Build history of the part. All positions in model axes, mm. A direction names the side the tool comes from. Give positions to 0.01 mm unless a question says otherwise; leave off trailing zeros. Order: outer loops, then holes, each group sorted by start corner. A loop starts at its lowest first (then second) coordinate and runs counter-clockwise, first axis right, second up. Notation, with made-up numbers: M -10.5,33.5 L 3.5,33.5 A25 cw 3.5,70.5 Z; hole C 1.5,29.5 d8. An arc over 180 degrees is marked long. One line per item, written item: value. Start each with the question number.
from build123d import *
from build123d.topology import SkipClean

# Parameters (mm, degrees)
SKETCH1_R               = 7.5
BOSS_EXTRUDE1_DEPTH     = 6.779166667
SKETCH1_3_R             = 7.5
BOSS_EXTRUDE2_DEPTH     = 2.779166667
BOSS_EXTRUDE3_START     = -4
SKETCH1_4_R             = 7.5
BOSS_EXTRUDE3_DEPTH     = 4
SKETCH2_R               = 5
BOSS_EXTRUDE4_DEPTH     = 6.016666667
SKETCH2_3_R             = 5.5
SKETCH2_3_R_2           = 5
BOSS_EXTRUDE5_DEPTH     = 1.254166667
BOSS_EXTRUDE9_START     = 16.541666667
SKETCH3_R               = 5
BOSS_EXTRUDE9_DEPTH     = 16.541666667
BOSS_EXTRUDE10_START    = 12.541666667
SKETCH3_3_R             = 5.5
SKETCH3_3_R_2           = 5
BOSS_EXTRUDE10_DEPTH    = 12.541666667
BOSS_EXTRUDE11_DEPTH    = 9.4
CUT_EXTRUDE1_DEPTH      = 28.502022969
CUT_EXTRUDE1_DEPTH_BACK = 28.502022969
SKETCH5_R               = 1.575
CUT_EXTRUDE5_START      = -2.779166667
CUT_EXTRUDE5_DEPTH      = 2.779166667
BOSS_EXTRUDE12_START    = -2.779166667
SKETCH6_4_R             = 9
BOSS_EXTRUDE12_DEPTH    = 2.779166667


with BuildPart() as part:
    # Sketch1 → Boss-Extrude1 (new body)
    with BuildSketch(Plane(origin=(0, 0, 0), x_dir=(1, 0, 0), z_dir=(0, 1, 0))):
        with Locations(Location((-1, 0, 0), (0, 0, 270))):
            Circle(SKETCH1_R)
    extrude(amount=BOSS_EXTRUDE1_DEPTH)

    # Sketch1<3> → Boss-Extrude2 (add)
    with BuildSketch(Plane(origin=(0, 0, 0), x_dir=(1, 0, 0), z_dir=(0, 1, 0))):
        with Locations(Location((-1, 0, 0), (0, 0, 82.337744339))):
            Circle(SKETCH1_3_R)
        with Locations((1, 0)):
            Circle(SKETCH1_3_R)
    extrude(amount=BOSS_EXTRUDE2_DEPTH)

    # Sketch1<4> → Boss-Extrude3 (add)
    with BuildSketch(Plane(origin=(0, 0, 0), x_dir=(1, 0, 0), z_dir=(0, 1, 0)).offset(BOSS_EXTRUDE3_START)):
        with Locations(Location((1, 0, 0), (0, 0, 97.662255661))):
            Circle(SKETCH1_4_R)
        with BuildLine():
            Line((-1.54175225, 2.127), (1.54175225, 2.127))
            ThreePointArc((1.54175225, 2.127), (0, -2.627), (-1.54175225, 2.127))
        make_face(mode=Mode.SUBTRACT)
    extrude(amount=BOSS_EXTRUDE3_DEPTH)

    # Sketch2 → Boss-Extrude4 (add)
    with BuildSketch(Plane.XZ.offset(4)):
        with Locations(Location((0, 0, 0), (0, 0, 90))):
            Circle(SKETCH2_R)
    extrude(amount=BOSS_EXTRUDE4_DEPTH)

    # Sketch2<3> → Boss-Extrude5 (add)
    with BuildSketch(Plane.XZ.offset(4)):
        with Locations(Location((0, 0, 0), (0, 0, 90))):
            Circle(SKETCH2_3_R)
        with Locations(Location((0, 0, 0), (0, 0, 270))):
            Circle(SKETCH2_3_R_2, mode=Mode.SUBTRACT)
    extrude(amount=BOSS_EXTRUDE5_DEPTH)

    # Sketch3 → Boss-Extrude9 (add)
    with BuildSketch(Plane(origin=(0, 6.779166667, 0), x_dir=(1, 0, 0), z_dir=(0, 1, 0)).offset(BOSS_EXTRUDE9_START)):
        with Locations(Location((0, 0, 0), (0, 0, 90))):
            Circle(SKETCH3_R)
    extrude(amount=-BOSS_EXTRUDE9_DEPTH)

    # Sketch3<3> → Boss-Extrude10 (add)
    with BuildSketch(Plane(origin=(0, 6.779166667, 0), x_dir=(1, 0, 0), z_dir=(0, 1, 0)).offset(BOSS_EXTRUDE10_START)):
        with Locations(Location((0, 0, 0), (0, 0, 270))):
            Circle(SKETCH3_3_R)
        with Locations(Location((0, 0, 0), (0, 0, 90))):
            Circle(SKETCH3_3_R_2, mode=Mode.SUBTRACT)
    extrude(amount=-BOSS_EXTRUDE10_DEPTH)

    # Sketch4 → Boss-Extrude11 (add)
    with BuildSketch(Plane.XZ.offset(10.016666667)):
        with BuildLine():
            Line((-4, 3), (-4, -3))
            ThreePointArc((-4, -3), (0, -5), (4, -3))
            Line((4, -3), (4, 3))
            ThreePointArc((4, 3), (0, 5), (-4, 3))
        make_face()
    extrude(amount=BOSS_EXTRUDE11_DEPTH)

    # Sketch5 → Cut-Extrude1 (cut, two sides: drawn at the far end of the back side and taken through both)
    with BuildSketch(Plane(origin=(4, 0, 0), x_dir=(0, 0, -1), z_dir=(1, 0, 0)).offset(-CUT_EXTRUDE1_DEPTH_BACK)):
        with Locations(Location((-1.35, -16.416666667, 0), (0, 0, 180))):
            Circle(SKETCH5_R)
        with Locations(Location((1.35, -13.416666667, 0), (0, 0, 180))):
            Circle(SKETCH5_R)
    extrude(amount=CUT_EXTRUDE1_DEPTH + CUT_EXTRUDE1_DEPTH_BACK, mode=Mode.SUBTRACT)

    # Sketch6 → Cut-Extrude5 (cut)
    with SkipClean():  # the faces are left unmerged after this step: merging them gives an invalid solid
        with BuildSketch(Plane(origin=(0, 2.779166667, 0), x_dir=(1, 0, 0), z_dir=(0, 1, 0)).offset(CUT_EXTRUDE5_START)):
            with BuildLine():
                ThreePointArc((0, -7.433034374), (8.5, 0), (0, 7.433034374))
                ThreePointArc((0, 7.433034374), (6.5, 0), (0, -7.433034374))
            make_face()
        extrude(amount=CUT_EXTRUDE5_DEPTH, mode=Mode.SUBTRACT)

    # Sketch6<4> → Boss-Extrude12 (add)
    # profile 1 of 2: a face of its own
    with BuildSketch(Plane(origin=(0, 2.779166667, 0), x_dir=(1, 0, 0), z_dir=(0, 1, 0)).offset(BOSS_EXTRUDE12_START)):
        with Locations(Location((0, 0, 0), (0, 0, 270))):
            Circle(SKETCH6_4_R)
        with BuildLine():
            ThreePointArc((0, 7.433034374), (6.5, 0), (0, -7.433034374))
            ThreePointArc((0, -7.433034374), (8.5, 0), (0, 7.433034374))
        make_face(mode=Mode.SUBTRACT)
    # profile 2 of 2: a face of its own
    with BuildSketch(Plane(origin=(0, 2.779166667, 0), x_dir=(1, 0, 0), z_dir=(0, 1, 0)).offset(BOSS_EXTRUDE12_START)):
        with BuildLine():
            ThreePointArc((0, -7.433034374), (8.5, 0), (0, 7.433034374))
            ThreePointArc((0, 7.433034374), (6.5, 0), (0, -7.433034374))
        make_face()
    extrude(amount=BOSS_EXTRUDE12_DEPTH)


solid = part.part
1) Slice it at A-A (y = -13). List the corners of the cut face in (x, z), plus the area to 3 significant figures.
2) Pull direction Z, two halves, no side cores. Call faces 5 (the cylindrical face through (2.703, 1.37, 8.584)), 6 (the flat face through (4, -15, 0)), 7 (the cylindrical face through (-0.056, -17.978, 1.145)): pulls with the +Z half, pulls with the -Z half, needs draft (parallel to the pull), parting line crosses it, or undercut.
3) Slice it at B-B (x = -1). State how many separate pieces and enclosed holes the cut face has, plus the area to 3 significant figures.
4) Drill centre lines: line 1 (X direction, y = -1.7, z = 0); line 2 (Y direction, x = -1.25, z = -1.35); line 3 (Y direction, x = 1.5, z = 1.25). Where is each one in solid material? Low to high.
5) Drop flat-ended pins along their axis: P1, Ø5, axis at x = -7, z = 1.5, coming from the -Y side; P2, Ø8, axis at x = 4, y = -11, coming from the +Z side; P3, Ø1.8, axis at y = -15, z = 0, coming from the +X side. Give the stop position or say it passes through.
6) Slice it at C-C (z = 4.25). List the corners of the cut face in (x, y).
7) Tool access for faces 1 (the cylindrical face through (0.092, -2.028, 2.625)), 2 (the cylindrical face through (8.473, -2.028, 0.635)), 3 (the flat face through (-4.9, 19.321, 1.6)), 4 (the flat face through (-4.4, -10.017, 0)): list every direction of +Z, -Z, +X, -X, +Y, -Y with a clear straight run to the whole face (end or side of a thin tool).
Results list:
1. outline: M -4,-3 A5 ccw 4,-3 L 4,-2.87 L -4,-2.87 Z; M -4,0.17 L 4,0.17 L 4,3 A5 ccw -4,3 Z
1. area: 46.1 mm²
2. face 5: parting line crosses it
2. face 6: needs draft
2. face 7: undercut
3. separate pieces: 1
3. enclosed holes: 3
3. area: 461 mm²
4. line 1: x = -6.5 to -2.63, 2.63 to 8.5
4. line 2: y = -19.42 to -14.99, -11.84 to -4, 0 to 23.32
4. line 3: y = -19.42 to -17.99, -14.84 to -4, 0 to 23.32
5. P1: stops at y = -10.02
5. P2: stops at z = 5
5. P3: stops at x = 4
6. outline: M -7.93,0 L -5.18,0 L -5.18,-4 L -3.49,-4 L -3.49,-5.25 L -2.63,-5.25 L -2.63,-19.42 L 2.63,-19.42 L 2.63,-5.25 L 3.49,-5.25 L 3.49,-4 L 7.18,-4 L 7.18,0 L 7.93,0 L 7.93,2.78 L 5.18,2.78 L 5.18,6.78 L 3.49,6.78 L 3.49,19.32 L 2.63,19.32 L 2.63,23.32 L -2.63,23.32 L -2.63,19.32 L -3.49,19.32 L -3.49,6.78 L -7.18,6.78 L -7.18,2.78 L -7.93,2.78 Z
7. face 1: none
7. face 2: -Y
7. face 3: +Y
7. face 4: +Z, -Z, -X, -Y
